Autodesk Inventor part; units mm, degrees
ref_plane "YZ Plane" through (0, 0, 0) normal (1, 0, 0) x (0, 1, 0)
ref_plane "XZ Plane" through (0, 0, 0) normal (0, 1, 0) x (-1, 0, 0)
ref_plane "XY Plane" through (0, 0, 0) normal (0, 0, 1) x (1, 0, 0)
sketch "Sketch1" plane through (0, 0, 0) normal (0, 0, 1) x (1, 0, 0)
  circle A0 centre (1.9895, 47.0752) radius 2
  line L0 (-3.9007, 3) -> (-3.9007, 30)
  line L1 (-3.9007, 40) -> (-3.9007, 55)
  circle A1 centre (1.9895, 47.0752) radius 5
  line L2 (1.9895, 47.0752) -> (-1.546, 43.5397)
  line L3 (1.9895, 47.0752) -> (6.9895, 47.0752) construction
  line L4 (1.9895, 47.0752) -> (5.525, 50.6108)
  arc A2 (1.9895, 1.5) -> (47.0122, 40) centre (1.9895, 47.0752) ccw
  arc A3 (1.9895, -1.5) -> (50.0467, 40) centre (1.9895, 47.0752) ccw
  line L5 (-1.546, 43.5397) -> (47.9514, -5.9578)
  line L6 (5.525, 50.6108) -> (55.0225, 1.1133)
  line L7 (47.9514, -5.9578) -> (55.0225, 1.1133)
  circle A4 centre (35.2767, 13.788) radius 1.5
  point P0 (0, 0)
  dimension "d0" = 10
  dimension "d1" = 135
  dimension "d3" = 10
  dimension "d4" = 3
  dimension "d5" = 5
  dimension "d6" = 70
extrude "Extrusion1" add sketch "Sketch1" along normal blind 4 contours A0 L2 L4 | A0 L4 A1 L2 | L4 L2 A0 | A0 L2 A1 L4 | L6 A2 L5 A1 | L6 A3 A4 A2 | A2 A4 A3 L5 | L6 L7 L5 A3
sketch "Sketch2" plane through (0, 0, 0) normal (0, 0, -1) x (-1, 0, 0)
  circle A0 centre (-1.9895, 47.0752) radius 2
  circle A1 centre (-1.9895, 47.0752) radius 1.85
  point P0 (0, 0)
  dimension "d9" = 3.7
extrude "Extrusion2" add sketch "Sketch2" along normal blind 4 contours A1
sketch "Sketch3" plane through (0, 0, 4) normal (0, 0, 1) x (1, 0, 0)
  circle A0 centre (35.2767, 13.788) radius 1.5
  arc A1 (5.525, 50.6108) -> (-1.546, 43.5397) centre (1.9895, 47.0752) ccw
  line L0 (-1.546, 43.5397) -> (47.9514, -5.9578)
  line L1 (47.9514, -5.9578) -> (55.0225, 1.1133)
  line L2 (55.0225, 1.1133) -> (5.525, 50.6108)
  circle A2 centre (46.5372, 2.5275) radius 1.5
  line L3 (35.2767, 13.788) -> (51.487, -2.4222)
  line L4 (47.9514, -5.9578) -> (55.0225, 1.1133)
  line L5 (55.0225, 1.1133) -> (5.525, 50.6108)
  point P0 (0, 0)
  dimension "d12" = 3
  dimension "d13" = 7
extrude "Extrusion3" cut sketch "Sketch3" against normal through all contours A2 L3 | L3 A2
properties part number "eye_tracker_angled_arm"
Can you work these out from the model? Positions are in its coordinate system, mm. A direction names the side the tool comes from. Round coordinates to 2 decimals unless told otherwise and drop trailing zeros. Loops run counter-clockwise (first coordinate to the right, second up) from the corner with the lowest first, then second, coordinate; pieces in that order, holes last. Notation, with made-up numbers: (63, -40) -> (112, -40) arc R29 cw to (112, -10) -> close; hole circle Ø4 at (-32, 42). An arc over 180 degrees is marked (long way). Answer in a Markdown table with one row per item.
Item 1: If I drill on probe 1 along Z at (x, y) = (45.5, 10); probe 2 along X at (y, z) = (3.5, 0.5); probe 3 along X at (y, z) = (13, 2.75), over which ranges is the centre line in solid material (lowest first)?
Answer block:
| item | result |
|---|---|
| probe 1 | 0 to 4 |
| probe 2 | 38.49 to 45.4, 47.68 to 52.64 |
| probe 3 | 28.99 to 34, 36.55 to 43.14 |
Item 2: Suppose I cut it at A-A, the plane x = 35.5. List the corners of the cut face in (y, z) for me, plus the area to 3 significant figures.
Answer block:
| item | result |
|---|---|
| outline | (6.49, 0) -> (12.3, 0) -> (12.3, 4) -> (6.49, 4) -> close; (15.27, 0) -> (20.64, 0) -> (20.64, 4) -> (15.27, 4) -> close |
| area | 44.7 mm² |
Item 3: Suppose I cut it at B-B, the plane x = 47. List the corners of the cut face in (y, z) for me, plus the area to 3 significant figures.
Answer block:
| item | result |
|---|---|
| outline | (-5.01, 0) -> (1.1, 0) -> (1.1, 4) -> (-5.01, 4) -> close; (3.95, 0) -> (9.14, 0) -> (9.14, 4) -> (3.95, 4) -> close |
| area | 45.2 mm² |
Item 4: Will this pin go through, and if not, where does the flat tip stop? P1, Ø12, axis at x = 23, y = 31.5, coming from the -Z side.
Answer block:
| item | result |
|---|---|
| P1 | z = 0 |
Item 5: Suppose I cut it at C-C, the plane y = 33.5. List the corners of the cut face in (x, z) for me, plus the area to 3 significant figures.
Answer block:
| item | result |
|---|---|
| outline | (8.49, 0) -> (22.64, 0) -> (22.64, 4) -> (8.49, 4) -> close |
| area | 56.6 mm² |
Item 6: We'd pull the mould along X, two halves only. Please class faces 3 (the cylindrical face through (34.086, 14.701, 1.972)), 4 (the cylindrical face through (-1.623, 50.532, 1.972)), 5 (the flat face through (22.856, 19.137, 1.972)), 6 (the flat face through (24, 25, 4)): released by +X, released by -X, zero draft, split by the parting line, or undercut.
Answer block:
| item | result |
|---|---|
| face 3 | undercut |
| face 4 | split by the parting line |
| face 5 | released by -X |
| face 6 | zero draft |
Item 7: On a 3-axis mill with a long thin cutter (end or side, diameter ignored), from which of +Z, -Z, +X, -X, +Y, -Y can I reach the whole of each face in a straight line? I mean faces 1 (the cylindrical face through (1.14, 48.72, -1.97)), 2 (the flat face through (29.927, 26.209, 1.972)). Say none if no direction works.
Answer block:
| item | result |
|---|---|
| face 1 | -Z |
| face 2 | +Z, -Z, +X, +Y |
Item 8: Suppose I cut it at D-D, the plane z = -3. List the corners of the cut face in (x, y) for me, plus the area to 3 significant figures.
Answer block:
| item | result |
|---|---|
| outline | circle Ø3.7 at (1.99, 47.08) |
| area | 10.8 mm² |
